Work out the finished part from the listing and answer in its coordinate system (mm). Give positions to 0.01 mm unless a question says otherwise; leave off trailing zeros. Loops run counter-clockwise (first coordinate to the right, second up) from the corner with the lowest first, then second, coordinate; pieces in that order, holes last. Notation, with made-up numbers: M 56,-7.5 L 95,-7.5 A29 cw 95,31.5 Z; hole C -39,78 d11. An arc over 180 degrees is marked long. Answer as a JSON object with one key per item and string values. Group by question number.
```python
from build123d import *

# Parameters (mm, degrees)
F1_DEPTH = 3
F2_R     = 5
F3_R     = 5
F4_R     = 5


with BuildPart() as f1:
    # F0 (on Front) → F1 (new body)
    with BuildSketch(Plane.XZ):
        Polygon((21.310295, -72.443289), (21.310295, 77.556711), (-108.689705, -72.443289), align=None)
    extrude(amount=F1_DEPTH)

    # F2
    f2_edges = [f1.edges().sort_by_distance(p)[0] for p in [
        (21.310295, -1.5, 77.556711),
    ]]
    fillet(f2_edges, radius=F2_R)

    # F3
    f3_edges = [f1.edges().sort_by_distance(p)[0] for p in [
        (21.310295, -1.5, -72.443289),
    ]]
    fillet(f3_edges, radius=F3_R)

    # F4
    f4_edges = [f1.edges().sort_by_distance(p)[0] for p in [
        (-108.689705, -1.5, -72.443289),
    ]]
    fillet(f4_edges, radius=F4_R)


solid = f1.part
```
Item 1: A cutting plane is placed at C-C (x = -25). Determine the outline of the cut face in (y, z).
Item 2: A cutting plane is placed at B-B (z = -42.5). Determine the outline of the cut face in (x, y).
Item 3: A cutting plane is placed at A-A (y = -1). Determine the outline of the cut face in (x, z), and give its area (3 significant figures).
Item 4: Find the intervals of material crossed by probe 1 along X at (y, z) = (-1.5, -45.5); probe 2 along X at (y, z) = (-0.95, 54.5); probe 3 along Z at (x, y) = (-95, -2.65), in increasing order. Write a range as [from, to].
The answers:
{
 "1": {"outline": "M -3,-72.44 L 0,-72.44 L 0,24.12 L -3,24.12 Z"},
 "2": {"outline": "M -82.74,-3 L 21.31,-3 L 21.31,0 L -82.74,0 Z"},
 "3": {"outline": "M -101.52,-64.17 A5 ccw -97.74,-72.44 L 16.31,-72.44 A5 ccw 21.31,-67.44 L 21.31,64.15 A5 ccw 12.53,67.43 Z", "area": "9,680 mm^2"},
 "4": {"probe 1": "x = [-85.34, 21.31]", "probe 2": "x = [1.33, 21.31]", "probe 3": "z = [-72.44, -56.65]"}
}
